```python
from build123d import *

# Parameters (mm, degrees)
SKETCH1_W           = 37
SKETCH1_H           = 15.3
BOSS_EXTRUDE1_DEPTH = 3
SKETCH2_W           = 34
SKETCH2_H           = 12
BOSS_EXTRUDE2_DEPTH = 1
SKETCH3_W           = 31
SKETCH3_H           = 10
CUT_EXTRUDE1_DEPTH  = 0.5
CUT_EXTRUDE2_DEPTH  = 5
SKETCH5_W           = 31
SKETCH5_H           = 12.5
BOSS_EXTRUDE3_DEPTH = 20


with BuildPart() as part:
    # Sketch1 → Boss-Extrude1 (new body)
    with BuildSketch(Plane(origin=(0, 0, 0), x_dir=(1, 0, 0), z_dir=(0, 1, 0))):
        Rectangle(SKETCH1_W, SKETCH1_H)
    extrude(amount=BOSS_EXTRUDE1_DEPTH)

    # Sketch2 → Boss-Extrude2 (add)
    with BuildSketch(Plane(origin=(0, 3, 0), x_dir=(1, 0, 0), z_dir=(0, 1, 0))):
        Rectangle(SKETCH2_W, SKETCH2_H)
    extrude(amount=BOSS_EXTRUDE2_DEPTH)

    # Sketch3 → Cut-Extrude1 (cut)
    with BuildSketch(Plane(origin=(0, 4, 0), x_dir=(1, 0, 0), z_dir=(0, 1, 0))):
        Rectangle(SKETCH3_W, SKETCH3_H)
    extrude(amount=-CUT_EXTRUDE1_DEPTH, mode=Mode.SUBTRACT)

    # Sketch4 → Cut-Extrude2 (cut)
    with BuildSketch(Plane(origin=(0, 3.5, 0), x_dir=(1, 0, 0), z_dir=(0, 1, 0))):
        with BuildLine():
            Line((-10.75, 3), (-9.75, 3))
            Line((-9.75, 3), (-9.75, 1.5))
            ThreePointArc((-9.75, 1.5), (-5.25, 0), (-9.75, -1.5))
            Line((-9.75, -1.5), (-9.75, -3))
            Line((-9.75, -3), (-10.75, -3))
            Line((-10.75, -3), (-10.75, 3))
        make_face()
        with BuildLine():
            Line((9.75, -1.5), (9.75, -3))
            Line((9.75, -3), (10.75, -3))
            Line((10.75, -3), (10.75, 3))
            Line((10.75, 3), (9.75, 3))
            Line((9.75, 3), (9.75, 1.5))
            ThreePointArc((9.75, 1.5), (5.25, 0), (9.75, -1.5))
        make_face()
    extrude(amount=-CUT_EXTRUDE2_DEPTH, mode=Mode.SUBTRACT)

    # Sketch5 → Boss-Extrude3 (add)
    with BuildSketch(Plane.XZ):
        Rectangle(SKETCH5_W, SKETCH5_H)
    extrude(amount=BOSS_EXTRUDE3_DEPTH)


solid = part.part
```
The listing builds one solid part. Answer for the finished solid, in the listing's coordinates (mm). A direction names the side the tool comes from. Coordinates: 2 decimals unless noted, no trailing zeros. Loops run counter-clockwise (first coordinate to the right, second up) from the corner with the lowest first, then second, coordinate; pieces in that order, holes last. Notation, with made-up numbers: (-11, -2) - (17, -2) arc R5 ccw to (17, 5) - close; hole circle Ø4 at (65.25, 30). An arc over 180 degrees is marked (long way). Write item = value, one per line.
1) Section C-C (x = -7.75) is taken. Determine the outline of the cut face in (y, z), plus the area to 3 significant figures.
Responses:
outline = (-20, -6.25) - (0, -6.25) - (0, -7.65) - (3, -7.65) - (3, -6) - (4, -6) - (4, -5) - (3.5, -5) - (3.5, -2.5) - (0, -2.5) - (0, 2.5) - (3.5, 2.5) - (3.5, 5) - (4, 5) - (4, 6) - (3, 6) - (3, 7.65) - (0, 7.65) - (0, 6.25) - (-20, 6.25) - close
area = 285 mm^2
2) Section A-A (y = 1.25) is taken. Determine the outline of the cut face in (x, z), plus the area to 3 significant figures.
Responses:
outline = (-18.5, -7.65) - (18.5, -7.65) - (18.5, 7.65) - (-18.5, 7.65) - close; hole (-10.75, -3) - (-9.75, -3) - (-9.75, -1.5) arc R2.5 ccw (long way) to (-9.75, 1.5) - (-9.75, 3) - (-10.75, 3) - close; hole (9.75, -3) - (10.75, -3) - (10.75, 3) - (9.75, 3) - (9.75, 1.5) arc R2.5 ccw (long way) to (9.75, -1.5) - close
area = 517 mm^2
3) Which of the six approach directions +Z, -Z, +X, -X, +Y, -Y give full straight-line access (tool end or side, diameter ignored) to faces 4 (the face through (-10, 2, -3)), 5 (the face through (0, -10, -6.25)), 6 (the face through (-0.2, 3.5, -6)), 7 (the face through (15.5, -10, 0)), 8 (the face through (18.5, 1, 0))?
Responses:
face_4 = +Y
face_5 = -Z, +X, -X, -Y
face_6 = -Z, +X, -X, +Y
face_7 = +Z, -Z, +X, -Y
face_8 = +Z, -Z, +X, +Y, -Y
4) Section B-B (z = 0) is taken. Determine the outline of the cut face in (x, y).
Responses:
outline = (-18.5, 0) - (-15.5, 0) - (-15.5, -20) - (15.5, -20) - (15.5, 0) - (18.5, 0) - (18.5, 3) - (17, 3) - (17, 4) - (15.5, 4) - (15.5, 3.5) - (10.75, 3.5) - (10.75, 0) - (5.25, 0) - (5.25, 3.5) - (-5.25, 3.5) - (-5.25, 0) - (-10.75, 0) - (-10.75, 3.5) - (-15.5, 3.5) - (-15.5, 4) - (-17, 4) - (-17, 3) - (-18.5, 3) - close
5) Find the intervals of material crossed by line 1 along X through (y, z) = (1.6, 0); line 2 along Z through (x, y) = (7.75, 2.6); line 3 along Z through (x, y) = (-3, -11), in increasing order.
Responses:
line_1 = -18.5 to -10.75, -5.25 to 5.25, 10.75 to 18.5
line_2 = -7.65 to -2.5, 2.5 to 7.65
line_3 = -6.25 to 6.25
6) Determine the mould class of faces 1 (the face through (-17, 3.5, 0.1)), 2 (the face through (-10, 2, 3)), 3 (the face through (0, -10, 6.25)) for opening direction Z: pulls with the +Z half, pulls with the -Z half, needs draft (parallel to the pull), parting line crosses it, or undercut.
Responses:
face_1 = needs draft
face_2 = undercut
face_3 = pulls with the +Z half
7) Each of these flat-tipped pins is pushed along its axis until it touches: P1, Ø1, axis at x = 11, y = -16.5, coming from the +Z side; P2, Ø1.5, axis at y = -15.5, z = -5.5, coming from the -X side; P3, Ø0.8, axis at x = -7, y = 3.5, coming from the +Z side. Where does it stop, or does it pass through?
Responses:
P1 = 6.25
P2 = -15.5
P3 = 6
8) Section D-D (x = -3) is taken. Determine the outline of the cut face in (y, z), plus the area to 3 significant figures.
Responses:
outline = (-20, -6.25) - (0, -6.25) - (0, -7.65) - (3, -7.65) - (3, -6) - (4, -6) - (4, -5) - (3.5, -5) - (3.5, 5) - (4, 5) - (4, 6) - (3, 6) - (3, 7.65) - (0, 7.65) - (0, 6.25) - (-20, 6.25) - close
area = 303 mm^2
